Input: part model. Units: mm. Frame: model coordinates. Coordinates: 2 decimals unless noted, no trailing zeros. Loops run counter-clockwise (first coordinate to the right, second up) from the corner with the lowest first, then second, coordinate; pieces in that order, holes last.
(1) Contact query for flat-ended pins moving along their axis: P1, Ø23.5, axis at x = -49.24, y = -14.24, coming from the -Z side; P2, Ø1.2, axis at x = -107.94, y = -28.39, coming from the +Z side. Output: stop coordinate, or through.
(2) Section C-C, the plane x = -69. Return loops of the section in (y, z), then the cut area to 3 significant figures.
(3) Section B-B, the plane y = 8. Return loops of the section in (x, z), then the cut area to 3 significant figures.
(4) Section A-A, the plane x = -8. Return loops of the section in (y, z).
(5) Line query: L1, parallel to X at y = -20, z = 1.7; L2, parallel to Y at x = 21, z = 1.65; L3, parallel to Y at x = -70.5, z = 1.8. Output: solid intervals per line, ascending.
(6) Section D-D, the plane z = 0.5. Give the number of separate pieces and of enclosed holes in the cut face, then the cut area to 3 significant figures.
```python
from build123d import *

# Parameters (mm, degrees)
SKETCH_1_R          = 3.05
SKETCH_1_R_2        = 5.05
EXTRUDE_1_DEPTH     = 2
SKETCH_2_R          = 3.05
CUT_EXTRUDE_1_DEPTH = 3.0000001
FILLET_1_R          = 10
FILLET_2_R          = 10
SKETCH_4_R          = 9
CUT_EXTRUDE_3_DEPTH = 10
FILLET_3_R          = 10
SKETCH_5_R          = 1
CUT_EXTRUDE_4_DEPTH = 10
CUT_EXTRUDE_5_DEPTH = 10


with BuildPart() as part:
    # 草图1 → 凸台-拉伸1 (new body)
    with BuildSketch(Plane.XY):
        with BuildLine():
            Line((33.781378488, 60.143481549), (26.111364219, 65.33671315))
            Line((26.111364219, 65.33671315), (-113.414892299, -28.455707895))
            Line((-113.414892299, -28.455707895), (-116.172277489, -83.735077284))
            ThreePointArc((-116.172277489, -83.735077284), (-103.256088302, -93.300423103), (-97.873109363, -78.156205675))
            Line((-97.873109363, -78.156205675), (-98.943047596, -76.564558134))
            Line((-98.943047596, -76.564558134), (51.562392304, 24.608295928))
            ThreePointArc((51.562392304, 24.608295928), (57.170026982, 19.385116489), (64.753479859, 20.488933768))
            add(Edge.make_bspline(
                [(64.753479859, 20.488933768), (66.638530957, 21.755918107), (68.426748806, 23.236531132), (70.062196414, 24.887697208)],
                knots=[0.026108887, 0.026108887, 0.026108887, 0.026108887, 0.973640222, 0.973640222, 0.973640222, 0.973640222], degree=3))
            ThreePointArc((70.062196414, 24.887697208), (78.287330396, 31.54858645), (87.76365302, 36.262351829))
            ThreePointArc((87.76365302, 36.262351829), (93.567944773, 44.696209097), (87.54263496, 52.973611636))
            ThreePointArc((87.54263496, 52.973611636), (79.818181838, 56.073118878), (72.738975332, 60.450213395))
            add(Edge.make_bspline(
                [(72.738975332, 60.450213395), (71.67095149, 61.35223039), (67.696722379, 64.109293298), (55.783849218, 67.566421953), (44.38146919, 64.224123675), (38.244385983, 60.128526636)],
                knots=[0.009949241, 0.009949241, 0.009949241, 0.009949241, 0.121591481, 0.393982167, 0.99006759, 0.99006759, 0.99006759, 0.99006759], degree=3))
            ThreePointArc((38.244385983, 60.128526636), (36.010602622, 59.45569692), (33.781378488, 60.143481549))
        make_face()
        with Locations((-106.172277489, -83.735077284)):
            Circle(SKETCH_1_R, mode=Mode.SUBTRACT)
        with Locations((59.811085021, 27.842354887)):
            Circle(SKETCH_1_R_2, mode=Mode.SUBTRACT)
    extrude(amount=EXTRUDE_1_DEPTH)

    # 草图2 → 切除-拉伸1 (cut, through all)
    with BuildSketch(Plane(origin=(0, 0, 0), x_dir=(-1, 0, 0), z_dir=(0, 0, -1))):
        with Locations((-84.708692938, 44.579039315)):
            Circle(SKETCH_2_R)
    extrude(amount=-CUT_EXTRUDE_1_DEPTH, mode=Mode.SUBTRACT)

    # 圆角1
    fillet_1_edges = [part.edges().sort_by_distance(p)[0] for p in [
        (51.562392304, 24.608295928, 1),
    ]]
    fillet(fillet_1_edges, radius=FILLET_1_R)

    # 圆角2
    fillet_2_edges = [part.edges().sort_by_distance(p)[0] for p in [
        (-113.414892299, -28.455707895, 1),
        (26.111364219, 65.33671315, 1),
    ]]
    fillet(fillet_2_edges, radius=FILLET_2_R)

    # 草图4 → 切除-拉伸3 (cut)
    with BuildSketch(Plane.XY.offset(2)):
        with Locations((-49.240629704, -14.235008927)):
            Circle(SKETCH_4_R)
        with Locations((-12.724289952, 10.312026151)):
            Circle(SKETCH_4_R)
        with Locations((23.792049801, 34.859061229)):
            Circle(SKETCH_4_R)
        with Locations((-85.756969456, -38.782044004)):
            Circle(SKETCH_4_R)
    extrude(amount=-CUT_EXTRUDE_3_DEPTH, mode=Mode.SUBTRACT)

    # 圆角3
    fillet_3_edges = [part.edges().sort_by_distance(p)[0] for p in [
        (-98.943047596, -76.564558134, 1),
    ]]
    fillet(fillet_3_edges, radius=FILLET_3_R)

    # 草图5 → 切除-拉伸4 (cut)
    with BuildSketch(Plane(origin=(0, 0, 0), x_dir=(-1, 0, 0), z_dir=(0, 0, -1))):
        with Locations((-22.674576674, 59.411613704)):
            Circle(SKETCH_5_R)
        with Locations((43.71876833, 14.780640835)):
            Circle(SKETCH_5_R)
        with Locations((107.944085943, -28.392939404)):
            Circle(SKETCH_5_R)
        with Locations((-46.10583743, 24.555107577)):
            Circle(SKETCH_5_R)
        with Locations((20.287507574, -20.075865292)):
            Circle(SKETCH_5_R)
        with Locations((74.553823436, -56.554799601)):
            Circle(SKETCH_5_R)
    extrude(amount=-CUT_EXTRUDE_4_DEPTH, mode=Mode.SUBTRACT)

    # 草图6 → 切除-拉伸5 (cut)
    with BuildSketch(Plane.XY.offset(2)):
        Polygon((4.648732698, 46.691800395), (6.322394181, 44.202049957), (-25.629403102, 22.723394264), (-27.303064585, 25.213144702), align=None)
        Polygon((-89.854720715, -20.450185975), (-57.902923432, 1.028469718), (-59.576584915, 3.518220156), (-91.528382198, -17.960435537), align=None)
    extrude(amount=-CUT_EXTRUDE_5_DEPTH, mode=Mode.SUBTRACT)


solid = part.part
```
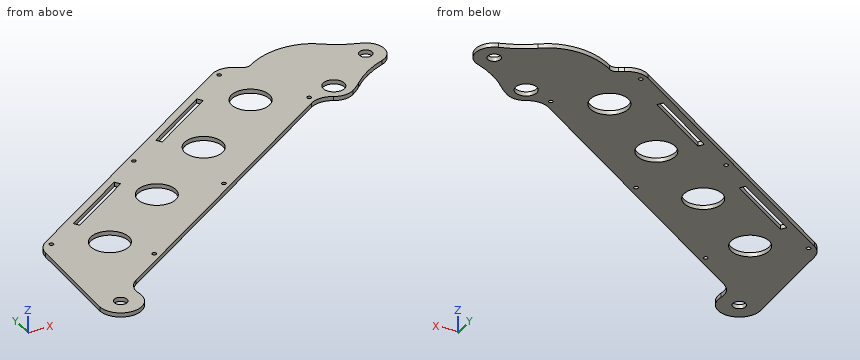
Report:
1. P1: stops at z = 0
1. P2: passes through
2. outline: (-56.44, 0) - (-6.43, 0) - (-6.43, 2) - (-56.44, 2) - close; (-2.82, 0) - (1.4, 0) - (1.4, 2) - (-2.82, 2) - close
2. area: 108 mm2
3. outline: (-59.18, 0) - (-21.42, 0) - (-21.42, 2) - (-59.18, 2) - close; (-4.03, 0) - (26.86, 0) - (26.86, 2) - (-4.03, 2) - close
3. area: 137 mm2
4. outline: (-15.43, 0) - (2.65, 0) - (2.65, 2) - (-15.43, 2) - close; (17.97, 0) - (34.57, 0) - (34.57, 2) - (17.97, 2) - close; (38.19, 0) - (42.41, 0) - (42.41, 2) - (38.19, 2) - close
5. L1: x = -100.84 to -90.16, -89.19 to -56.15, -42.33 to -21.28, -19.29 to -14.8
5. L2: y = 4.06 to 26.3, 43.42 to 61.88
5. L3: y = -57.44 to -7.44, -3.82 to 0.39
6. separate pieces: 1
6. enclosed holes: 15
6. area: 9,480 mm2
